Verification items for this drawing (mm, ordinates from the low corner). Give positions to 0.01 mm unless a question says otherwise; leave off trailing zeros. Loops run counter-clockwise (first coordinate to the right, second up) from the corner with the lowest first, then second, coordinate; pieces in that order, holes last. Notation, with made-up numbers: (9.5, -8.75) -> (21.5, -8.75) arc R19 ccw to (21.5, 11.25) -> close; hole circle Ø4 at (76, 46). An arc over 180 degrees is marked (long way). Write item = value, one per line.
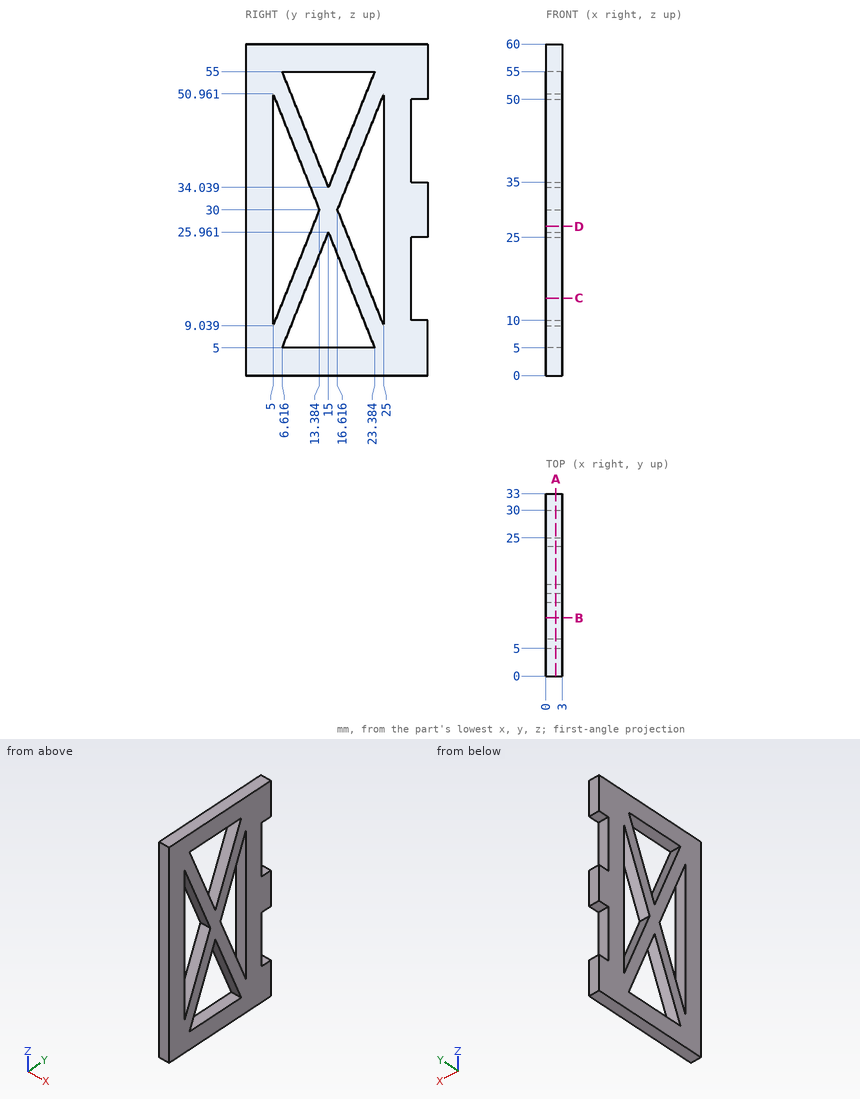
Item 1: Section check C-C, the plane z = 14. Record the cut outline in (x, y) (1 decimal).
Answer:
outline = (0, 0) -> (3, 0) -> (3, 5) -> (0, 5) -> close; (0, 7) -> (3, 7) -> (3, 10.2) -> (0, 10.2) -> close; (0, 19.8) -> (3, 19.8) -> (3, 23) -> (0, 23) -> close; (0, 25) -> (3, 25) -> (3, 30) -> (0, 30) -> close
Item 2: Section check D-D, the plane z = 27. Record the cut outline in (x, y) (1 decimal).
Answer:
outline = (0, 0) -> (3, 0) -> (3, 5) -> (0, 5) -> close; (0, 12.2) -> (3, 12.2) -> (3, 17.8) -> (0, 17.8) -> close; (0, 25) -> (3, 25) -> (3, 33) -> (0, 33) -> close
Item 3: Gauge pin test, flat end, axial feed: pin 1 (1.5 mm diameter, centred on x = 1.5, z = 40, fed in from +Y). Record the tip position at first contact, or that the pin passes through.
Answer:
pin_1 = 30
Item 4: Section check B-B, the plane y = 10.5. Record the cut outline in (x, z).
Answer:
outline = (0, 0) -> (3, 0) -> (3, 5) -> (0, 5) -> close; (0, 14.71) -> (3, 14.71) -> (3, 22.79) -> (0, 22.79) -> close; (0, 37.21) -> (3, 37.21) -> (3, 45.29) -> (0, 45.29) -> close; (0, 55) -> (3, 55) -> (3, 60) -> (0, 60) -> close
Item 5: Thickness scan on L1, parallel to Z at x = 0.35, y = 31.5; L2, parallel to Y at x = 0.6, z = 23 (1 decimal); L3, parallel to Y at x = 0.6, z = 17.5 (1 decimal). Record the ranges inside material, lowest first. Write a range as [from, to].
Answer:
L1 = [0, 10], [25, 35], [50, 60]
L2 = [0, 5], [10.6, 13.8], [16.2, 19.4], [25, 30]
L3 = [0, 5], [8.4, 11.6], [18.4, 21.6], [25, 30]
Item 6: Section check A-A, the plane x = 1.8. Record the cut outline in (y, z) (1 decimal), plus the area to 3 significant figures.
Answer:
outline = (0, 0) -> (33, 0) -> (33, 10) -> (30, 10) -> (30, 25) -> (33, 25) -> (33, 35) -> (30, 35) -> (30, 50) -> (33, 50) -> (33, 60) -> (0, 60) -> close; hole (5, 9) -> (13.4, 30) -> (5, 51) -> close; hole (6.6, 5) -> (23.4, 5) -> (15, 26) -> close; hole (6.6, 55) -> (15, 34) -> (23.4, 55) -> close; hole (16.6, 30) -> (25, 9) -> (25, 51) -> close
area = 1,190 mm^2
